Geometry check sheet. Reference: drawing and pictorial views, mm from the part's lowest x, y, z. Round coordinates to 2 decimals unless told otherwise and drop trailing zeros. Write each loop counter-clockwise with the first axis right and the second up, starting at its lowest first coordinate (ties: lowest second). Pieces come first, ordered by that corner, then holes.
Item 1: Section check B-B, the plane y = 32. Record the cut outline in (x, z), plus the area to 3 significant figures.
Item 2: Section check A-A, the plane z = 10. Record the cut outline in (x, y), plus the area to 3 significant figures.
Item 3: Section check D-D, the plane y = 20. Record the cut outline in (x, z).
Item 4: Material ranges on line 1 along Y through (x, z) = (4, 15.75); line 2 along Z through (x, y) = (3, 8); line 3 along Y through (x, z) = (5.5, 10), recorded low to high.
Item 5: Release check for a two-part mould opening along Z. For the marked faces 1, 2, 3 and 4 record: pulls with the +Z half, pulls with the -Z half, needs draft (parallel to the pull), parting line crosses it, or undercut.
Item 6: Depth check by flat-ended pin: pin 1 (2 mm diameter, centred on y = 8, z = 10, fed in from -X); pin 2 (10 mm diameter, centred on y = 10.5, z = 15, fed in from -X). Enter the tip coordinate at first touch or a pass-through.
Item 7: Section check C-C, the plane x = 4.25. Record the cut outline in (y, z).
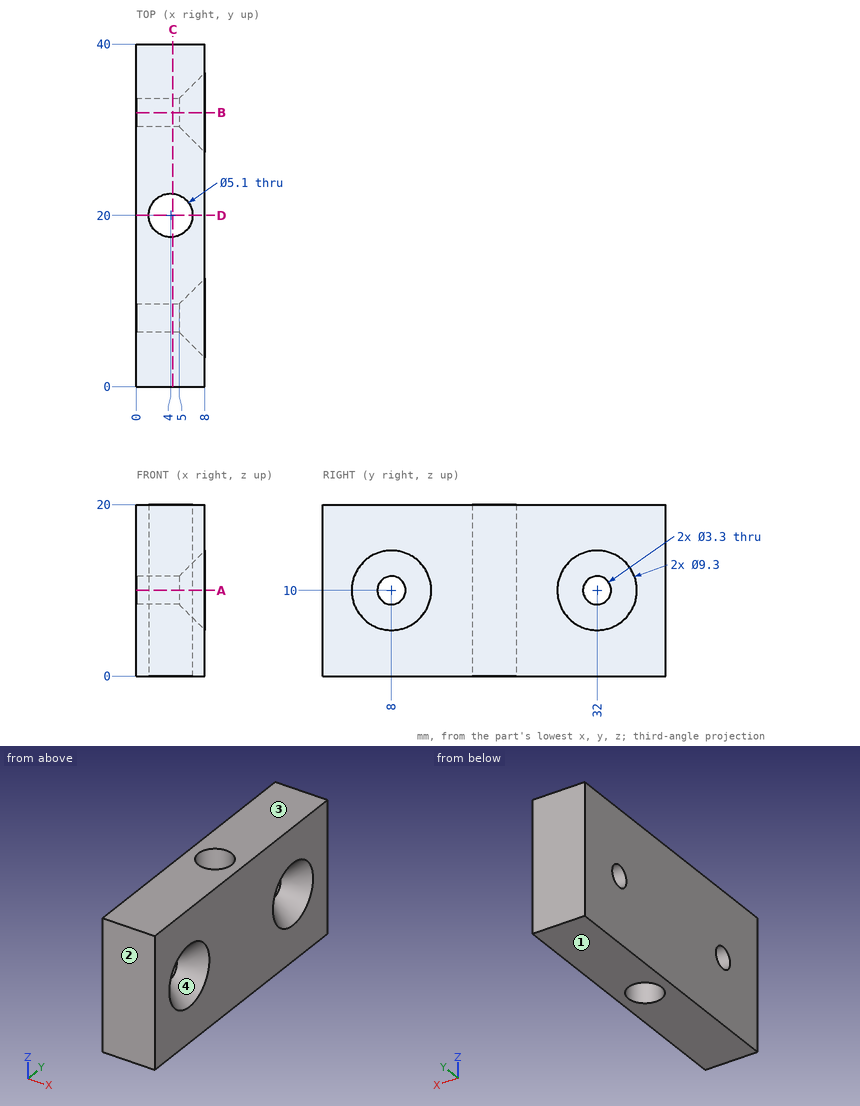
Values found:
1. outline: (0, 0) - (8, 0) - (8, 5.35) - (5, 8.35) - (0, 8.35) - close; (0, 11.65) - (5, 11.65) - (8, 14.65) - (8, 20) - (0, 20) - close
1. area: 125 mm2
2. outline: (0, 0) - (8, 0) - (8, 3.35) - (5, 6.35) - (0, 6.35) - close; (0, 9.65) - (5, 9.65) - (8, 12.65) - (8, 27.35) - (5, 30.35) - (0, 30.35) - close; (0, 33.65) - (5, 33.65) - (8, 36.65) - (8, 40) - (0, 40) - close; hole circle Ø5.1 at (4, 20)
2. area: 229 mm2
3. outline: (0, 0) - (1.45, 0) - (1.45, 20) - (0, 20) - close; (6.55, 0) - (8, 0) - (8, 20) - (6.55, 20) - close
4. line 1: y = 0 to 17.45, 22.55 to 40
4. line 2: z = 0 to 8.35, 11.65 to 20
4. line 3: y = 0 to 5.85, 10.15 to 17.94, 22.06 to 29.85, 34.15 to 40
5. face 1: pulls with the -Z half
5. face 2: needs draft
5. face 3: pulls with the +Z half
5. face 4: undercut
6. pin 1: passes through
6. pin 2: stops at x = 0
7. outline: (0, 0) - (17.46, 0) - (17.46, 20) - (0, 20) - close; (22.54, 0) - (40, 0) - (40, 20) - (22.54, 20) - close; hole circle Ø3.3 at (8, 10); hole circle Ø3.3 at (32, 10)
